from build123d import *

# Parameters (mm, degrees)
F0_W      = 76.2000009418
F0_H      = 56.3335753977
F1_DEPTH  = 50.8
F2_W      = 61.2327515673
F2_H      = 46.8085720204
F3_DEPTH  = 43.18
F4_W      = 46.8085720204
F4_H      = 21.59
F5_DEPTH  = 25.4
F6_W      = 46.8085720204
F6_H      = 9.227910161
F7_DEPTH  = 25.4
F9_DEPTH  = 5.08
F10_R     = 1.524
F11_DEPTH = 25.4
F12_W     = 46.8085720204
F12_H     = 5.665987947
F13_DEPTH = 25.4


with BuildPart() as f1:
    # F0 (on Top) → F1 (new body)
    with BuildSketch(Plane.XY):
        with Locations((38.1000004709, -28.1667876989)):
            Rectangle(F0_W, F0_H)
    extrude(amount=F1_DEPTH)

    # F2 (on face) → F3 (cut)
    with BuildSketch(Plane.XY.offset(50.8)):
        with Locations((38.5085178336, -27.7585715521)):
            Rectangle(F2_W, F2_H)
    extrude(amount=-F3_DEPTH, mode=Mode.SUBTRACT)

    # F4 (on face) → F5 (cut)
    with BuildSketch(Plane.YZ.offset(7.89214205)):
        with Locations((-27.7585715521, 18.415)):
            Rectangle(F4_W, F4_H)
    extrude(amount=-F5_DEPTH, mode=Mode.SUBTRACT)

    # F6 (on face) → F7 (cut)
    with BuildSketch(Plane(origin=(0, 0, 0), x_dir=(0, -1, 0), z_dir=(-1, 0, 0))):
        with Locations((27.7585715521, 33.8239550805)):
            Rectangle(F6_W, F6_H)
    extrude(amount=-F7_DEPTH, mode=Mode.SUBTRACT)

    # F8 (on face) → F9 (cut)
    with BuildSketch(Plane.XY.offset(7.62)):
        Polygon((26.1257160455, -9.5250001177), (26.1257160455, -16.6007149965), (26.1257160455, -37.2835732996), (33.4735698998, -37.2835732996), (33.4735698998, -27.7585722506), (40.821429342, -37.2835732996), (46.1298863749, -33.1884770438), (37.9123979826, -22.5361794362), (46.1298863749, -16.1969728194), (42.6624452598, -11.7021426558), (33.4735698998, -17.097555101), (33.4735698998, -9.5250001177), align=None)
    extrude(amount=-F9_DEPTH, mode=Mode.SUBTRACT)

    # F10 (on face) → F11 (cut)
    with BuildSketch(Plane.YZ.offset(76.2000009418)):
        with Locations((-44.9035726488, 18.5057148337)):
            Circle(F10_R)
        with Locations((-13.6071434245, 40.0050021708)):
            Circle(F10_R)
        with Locations((-44.9035726488, 40.0050021708)):
            Circle(F10_R)
        with Locations((-13.6071434245, 18.5057148337)):
            Circle(F10_R)
    extrude(amount=-F11_DEPTH, mode=Mode.SUBTRACT)

    # F12 (on face) → F13 (cut)
    with BuildSketch(Plane(origin=(0, 0, 0), x_dir=(0, -1, 0), z_dir=(-1, 0, 0))):
        with Locations((27.7585715521, 41.2709041345)):
            Rectangle(F12_W, F12_H)
    extrude(amount=-F13_DEPTH, mode=Mode.SUBTRACT)


solid = f1.part
Part model, mm, in its own coordinate system. A direction names the side the tool comes from. Round coordinates to 2 decimals unless told otherwise and drop trailing zeros. Order: outer loops, then holes, each group sorted by start corner. A loop starts at its lowest first (then second) coordinate and runs counter-clockwise, first axis right, second up. Notation, with made-up numbers: (-28.75, 35.5) -> (6.25, 35.5) arc R35 cw to (6.25, 72.5) -> close; hole circle Ø9 at (-17, 23). An arc over 180 degrees is marked (long way). Put each result on its own line as item: value.
Q1. Pin check, flat tips, straight feed: pin 1 Ø10 at (y, z) = (-29.5, 40) entering from -X; pin 2 Ø8 at (x, y) = (19.5, -46.5) entering from +Z; pin 3 Ø2.5 at (y, z) = (-44.9, 18.51) entering from +X; pin 4 Ø4 at (y, z) = (-13.61, 40.01) entering from -X. Stop position of each tip, or through.
From the geometry:
pin 1: stops at x = 0
pin 2: stops at z = 7.62
pin 3: passes through
pin 4: stops at x = 69.12
Q2. Band-saw the part on C-C (x = 24). Give the cut face in (y, z).
From the geometry:
outline: (-56.33, 0) -> (0, 0) -> (0, 50.8) -> (-4.35, 50.8) -> (-4.35, 7.62) -> (-51.16, 7.62) -> (-51.16, 50.8) -> (-56.33, 50.8) -> close
Q3. Wall check: line 1 (Y direction, x = 42, z = 22.5); line 2 (Z direction, x = 26.5, y = -51); line 3 (X direction, y = -5, z = 15). Give the ranges that are in metal, low to high. Write a range as [from, to].
From the geometry:
line 1: y = [-56.33, -51.16], [-4.35, 0]
line 2: z = [0, 7.62]
line 3: x = [69.12, 76.2]
Q4. Band-saw the part on D-D (z = 46.5). Give the cut face in (x, y), and give its area (3 significant figures).
From the geometry:
outline: (0, -56.33) -> (76.2, -56.33) -> (76.2, 0) -> (0, 0) -> close; hole (7.89, -51.16) -> (69.12, -51.16) -> (69.12, -4.35) -> (7.89, -4.35) -> close
area: 1,430 mm2
Q5. Tool access for faces 4 (the face through (30, -37.284, 5)), 5 (the face through (4, -27, 44.104)), 6 (the face through (72.71, -15.13, 40.07)): list every direction of +Z, -Z, +X, -X, +Y, -Y with a clear straight run to the whole face (end or side of a thin tool).
From the geometry:
face 4: +Z
face 5: -X
face 6: +X, -X
Q6. Band-saw the part on A-A (y = -41.5). Give the cut face in (x, z).
From the geometry:
outline: (0, 0) -> (76.2, 0) -> (76.2, 50.8) -> (69.12, 50.8) -> (69.12, 7.62) -> (0, 7.62) -> close; (0, 44.1) -> (7.89, 44.1) -> (7.89, 50.8) -> (0, 50.8) -> close
Q7. Band-saw the part on B-B (z = 15.5). Give the cut face in (x, y).
From the geometry:
outline: (0, -56.33) -> (76.2, -56.33) -> (76.2, 0) -> (0, 0) -> (0, -4.35) -> (69.12, -4.35) -> (69.12, -51.16) -> (0, -51.16) -> close
Q8. Pull direction X, two halves, no side cores. Call faces 1 (the face through (72.7, -44.1, 41.3)), 2 (the face through (30, -9.525, 5)), 3 (the face through (76.2, -29, 25)): pulls with the +X half, pulls with the -X half, needs draft (parallel to the pull), parting line crosses it, or undercut.
From the geometry:
face 1: needs draft
face 2: undercut
face 3: pulls with the +X half
